Could you check a few things on this model? Use its own coordinates, in mm. Face numbers are marked on the shaded views. Coordinates: 2 decimals unless noted, no trailing zeros. Write each loop counter-clockwise with the first axis right and the second up, starting at its lowest first coordinate (ties: lowest second). Pieces come first, ordered by that corner, then holes. Notation, with made-up numbers: (11.5, 73) - (47.5, 73) arc R21 cw to (47.5, 78) - close; hole circle Ø4 at (-17.5, 76.25). An arc over 180 degrees is marked (long way). Answer as a JSON object with one key per item and string values. Group by question number.
1) If we section it at B-B (z = 3): Write out the boundary of the cut face in (x, y), plus the area to 3 significant figures.
2) If we section it at D-D (y = 9): Write out the boundary of the cut face in (x, z).
3) If we section it at C-C (y = 43.5): Write out the boundary of the cut face in (x, z), plus the area to 3 significant figures.
4) Please list where these lines run through material, in increasing order: line 1 along X through (y, z) = (12, 2.75); line 2 along X through (y, z) = (26.5, 0.5); line 3 along X through (y, z) = (65, 0.5).
5) Will these pins go through, and if not, where does the flat tip stop? pin 1 Ø1.6 at (x, z) = (-15.5, -1.5) entering from -Y; pin 2 Ø8 at (x, y) = (10.5, -9) entering from -Z; pin 3 Ø4 at (x, y) = (17, 8.5) entering from -Z; pin 4 Ø0.9 at (y, z) = (33, -2) entering from -X.
6) If we section it at A-A (y = -2.5): Write out the boundary of the cut face in (x, z), plus the area to 3 significant figures.
7) We'd pull the mould along X, two halves only. Please class the marked faces 1 and 2: released by +X, released by -X, zero draft, split by the parting line, or undercut.
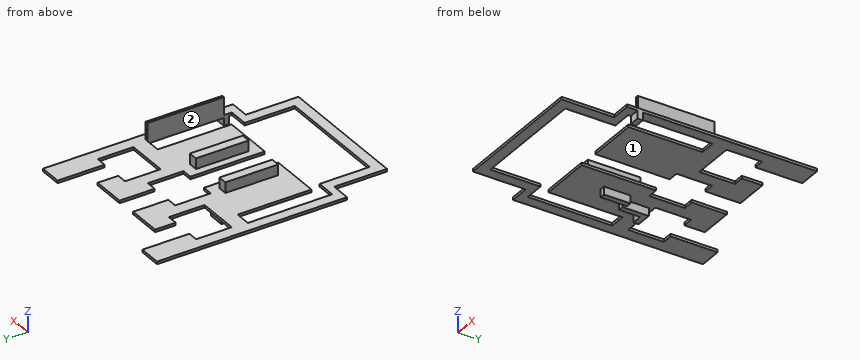
```python
from build123d import *

# Parameters (mm, degrees)
BOSS_EXTRUDE1_DEPTH = 1
SKETCH2_W           = 16
SKETCH2_H           = 13.5
CUT_EXTRUDE2_DEPTH  = 1
SKETCH5_W           = 1
SKETCH5_H           = 29
BOSS_EXTRUDE3_DEPTH = 6.75
SKETCH6_W           = 3.5
SKETCH6_H           = 20
BOSS_EXTRUDE4_DEPTH = 4
SKETCH7_W           = 4
SKETCH7_H           = 2
SKETCH7_W_2         = 2
SKETCH7_H_2         = 10
BOSS_EXTRUDE5_DEPTH = 3


with BuildPart() as part:
    # Sketch1 → Boss-Extrude1 (new body)
    with BuildSketch(Plane.XY):
        Polygon((0, 0), (0, 72), (-33.5, 72), (-33.5, 0), (-26, 0), align=None)
        Polygon((26, 0), (33.5, 0), (33.5, 72), (0, 72), (0, 0), align=None)
        Polygon((26, -20), (26, 0), (0, 0), (-26, 0), (-26, -20), align=None)
    extrude(amount=BOSS_EXTRUDE1_DEPTH)

    # Sketch2 → Cut-Extrude2 (cut)
    with BuildSketch(Plane.XY.offset(1)):
        Polygon((22, -16), (-22, -16), (-22, 3), (-29.5, 3), (-29.5, 35), (-23.5, 35), (-23.5, 7), (-4, 7), (-4, 35.2), (-8, 35.2), (-8, 48.7), (-4, 48.7), (-4, 62), (-16.9, 62), (-16.9, 54.2), (-24.9, 54.2), (-24.9, 72), (-16.9, 72), (16.9, 72), (24.9, 72), (24.9, 54.2), (16.9, 54.2), (16.9, 62), (4, 62), (4, 48.7), (8, 48.7), (8, 35.2), (4, 35.2), (4, 7), (23.5, 7), (23.5, 35), (29.5, 35), (29.5, 3), (22, 3), align=None)
        with Locations((20.9, 47.45)):
            Rectangle(SKETCH2_W, SKETCH2_H)
        with Locations((-20.9, 47.45)):
            Rectangle(SKETCH2_W, SKETCH2_H)
    extrude(amount=-CUT_EXTRUDE2_DEPTH, mode=Mode.SUBTRACT)

    # Sketch5 → Boss-Extrude3 (add)
    with BuildSketch(Plane.XY.offset(1)):
        with Locations((30, 20.5)):
            Rectangle(SKETCH5_W, SKETCH5_H)
    extrude(amount=BOSS_EXTRUDE3_DEPTH)

    # Sketch6 → Boss-Extrude4 (add)
    with BuildSketch(Plane.XY.offset(1)):
        with Locations((8.65, 21.2)):
            Rectangle(SKETCH6_W, SKETCH6_H)
    boss_extrude4 = extrude(amount=BOSS_EXTRUDE4_DEPTH)

    # Mirror1: Boss-Extrude4 across plane
    add(boss_extrude4.mirror(Plane(origin=(0, 0, 0), x_dir=(0, 0, 1), z_dir=(1, 0, 0))))

    # Sketch7 → Boss-Extrude5 (add)
    with BuildSketch(Plane(origin=(0, 0, 0), x_dir=(-1, 0, 0), z_dir=(0, 0, -1))):
        Polygon((14.2, 29), (16.2, 29), (16.2, 37), (20.2, 37), (20.2, 39), (16.2, 39), (14.2, 39), align=None)
        with Locations((-31.5, 5)):
            Rectangle(SKETCH7_W, SKETCH7_H)
        with Locations((12, 25)):
            Rectangle(SKETCH7_W_2, SKETCH7_H_2)
    extrude(amount=BOSS_EXTRUDE5_DEPTH)


solid = part.part
```
Here are the results:
{
 "1": {"outline": "(-10.4, 11.2) - (-6.9, 11.2) - (-6.9, 31.2) - (-10.4, 31.2) - close; (6.9, 11.2) - (10.4, 11.2) - (10.4, 31.2) - (6.9, 31.2) - close; (29.5, 6) - (30.5, 6) - (30.5, 35) - (29.5, 35) - close", "area": "169 mm²"},
 "2": {"outline": "(-33.5, 0) - (-29.5, 0) - (-29.5, 1) - (-33.5, 1) - close; (-23.5, 0) - (-4, 0) - (-4, 1) - (-23.5, 1) - close; (4, 0) - (23.5, 0) - (23.5, 1) - (4, 1) - close; (29.5, 0) - (33.5, 0) - (33.5, 1) - (30.5, 1) - (30.5, 7.75) - (29.5, 7.75) - close"},
 "3": {"outline": "(-33.5, 0) - (-28.9, 0) - (-28.9, 1) - (-33.5, 1) - close; (-12.9, 0) - (-8, 0) - (-8, 1) - (-12.9, 1) - close; (8, 0) - (12.9, 0) - (12.9, 1) - (8, 1) - close; (28.9, 0) - (33.5, 0) - (33.5, 1) - (28.9, 1) - close", "area": "19.0 mm²"},
 "4": {"line 1": "x = -10.4 to -6.9, 6.9 to 10.4, 29.5 to 30.5", "line 2": "x = -33.5 to -29.5, -23.5 to -4, 4 to 23.5, 29.5 to 33.5", "line 3": "x = -33.5 to -24.9, 24.9 to 33.5"},
 "5": {"pin 1": "stops at y = 29", "pin 2": "passes through", "pin 3": "stops at z = 0", "pin 4": "stops at x = -16.2"},
 "6": {"outline": "(-26, 0) - (-22, 0) - (-22, 1) - (-26, 1) - close; (22, 0) - (26, 0) - (26, 1) - (22, 1) - close", "area": "8.00 mm²"},
 "7": {"face 1": "zero draft", "face 2": "undercut"}
}
